Here's how the part is built. I have some questions about the finished solid (model axes, mm). A direction names the side the tool comes from. Round coordinates to 2 decimals unless told otherwise and drop trailing zeros. Write each loop counter-clockwise with the first axis right and the second up, starting at its lowest first coordinate (ties: lowest second). Pieces come first, ordered by that corner, then holes. Notation, with made-up numbers: (61.25, 26.25) -> (118.25, 26.25) arc R22 cw to (118.25, 58.25) -> close; hole circle Ø6 at (29, -40). An arc over 180 degrees is marked (long way). Answer as CSV lines item,"result".
```python
from build123d import *

# Parameters (mm, degrees)
F0_W     = 215.9
F0_H     = 63.5
F1_DEPTH = 19.05
F2_W     = 9.525
F2_H     = 50.8
F3_DEPTH = 25.4
F4_W     = 9.525
F4_H     = 50.8
F5_DEPTH = 25.4


with BuildPart() as f1:
    # F0 (on Right) → F1 (new body)
    with BuildSketch(Plane.YZ):
        with Locations((0, -31.75)):
            Rectangle(F0_W, F0_H)
    extrude(amount=F1_DEPTH)

    # F2 (on face) → F3 (join)
    with BuildSketch(Plane(origin=(0, 107.95, 0), x_dir=(-1, 0, 0), z_dir=(0, 1, 0))):
        with Locations((-9.525, -31.75)):
            Rectangle(F2_W, F2_H)
    extrude(amount=F3_DEPTH)

    # F4 (on face) → F5 (join)
    with BuildSketch(Plane.XZ.offset(107.95)):
        with Locations((9.525, -31.75)):
            Rectangle(F4_W, F4_H)
    extrude(amount=F5_DEPTH)


solid = f1.part
```
1. Suppose I cut it at A-A on z = -45. Please give me the cut outline in (x, y), and give its area (3 significant figures).
Numbers:
outline,"(0, -107.95) -> (4.76, -107.95) -> (4.76, -133.35) -> (14.29, -133.35) -> (14.29, -107.95) -> (19.05, -107.95) -> (19.05, 107.95) -> (14.29, 107.95) -> (14.29, 133.35) -> (4.76, 133.35) -> (4.76, 107.95) -> (0, 107.95) -> close"
area,"4,600 mm^2"
2. On a 3-axis mill with a long thin cutter (end or side, diameter ignored), from which of +Z, -Z, +X, -X, +Y, -Y can I reach the whole of each face in a straight line? I mean faces 1 (the face through (4.762, -120, -32)), 2 (the face through (14.288, 120, -32)), 3 (the face through (10, 120, -57.15)). Say none if no direction works.
Numbers:
face 1,"+Z, -Z, -X, -Y"
face 2,"+Z, -Z, +X, +Y"
face 3,"-Z, +X, -X, +Y"
3. Suppose I cut it at B-B on x = 11.5. Please give me the cut outline in (y, z), and give its area (3 significant figures).
Numbers:
outline,"(-133.35, -57.15) -> (-107.95, -57.15) -> (-107.95, -63.5) -> (107.95, -63.5) -> (107.95, -57.15) -> (133.35, -57.15) -> (133.35, -6.35) -> (107.95, -6.35) -> (107.95, 0) -> (-107.95, 0) -> (-107.95, -6.35) -> (-133.35, -6.35) -> close"
area,"16,300 mm^2"
4. For pin 1 Ø1.5 at (x, y) = (16.5, -19.5) entering from +Z; pin 2 Ø10.5 at (x, y) = (9, -121.5) entering from -Z; pin 3 Ø3 at (x, y) = (10.5, -126) entering from +Z; pin 4 Ø20.5 at (y, z) = (-125.5, -37.5) entering from -X, each with a flat end and sliding along its axis, tell me the tip position at first contact or that it passes through.
Numbers:
pin 1,"stops at z = 0"
pin 2,"stops at z = -57.15"
pin 3,"stops at z = -6.35"
pin 4,"stops at x = 4.76"
5. If I drill on line 1 (Y direction, x = 4, z = -4.5); line 2 (Z direction, x = 10.25, y = 122); line 3 (X direction, y = 112.5, z = -39), over which ranges is the centre line in solid material (lowest first)?
Numbers:
line 1,"y = -107.95 to 107.95"
line 2,"z = -57.15 to -6.35"
line 3,"x = 4.76 to 14.29"
